```python
from build123d import *

# Parameters (mm, degrees)
SKIZZE1_W                                      = 100
SKIZZE1_H                                      = 70
SKIZZE1_W_2                                    = 55
SKIZZE1_H_2                                    = 10
AUFSATZ_LINEAR_AUSTRAGEN1_DEPTH                = 2
F_3_5_3_5_DURCHMESSER_BOHRUNG1_D               = 3.5
FORMSENKUNG_F_R_M3_LINSENSENKSCHRAUB_2_COUNT   = 2
FORMSENKUNG_F_R_M3_LINSENSENKSCHRAUB_2_PITCH   = 90
FORMSENKUNG_F_R_M3_LINSENSENKSCHRAUB_3_COUNT   = 2
FORMSENKUNG_F_R_M3_LINSENSENKSCHRAUB_3_PITCH   = 108.166538264
FORMSENKUNG_F_R_M3_LINSENSENKSCHRAUB_4_COUNT   = 2
FORMSENKUNG_F_R_M3_LINSENSENKSCHRAUB_4_PITCH   = 60
FORMSENKUNG_F_R_M3_LINSENSENKSCHRAUB_5_A_COUNT = 2
FORMSENKUNG_F_R_M3_LINSENSENKSCHRAUB_5_A_PITCH = 20


with BuildPart() as part:
    # Skizze1 → Aufsatz-Linear austragen1 (new body)
    with BuildSketch(Plane(origin=(0, 0, 0), x_dir=(1, 0, 0), z_dir=(0, 1, 0))):
        with Locations((50, 35)):
            Rectangle(SKIZZE1_W, SKIZZE1_H)
        with Locations((37.5, 55)):
            Rectangle(SKIZZE1_W_2, SKIZZE1_H_2, mode=Mode.SUBTRACT)
    extrude(amount=AUFSATZ_LINEAR_AUSTRAGEN1_DEPTH)

    # Ø3.5 (3.5) Durchmesser Bohrung1 (through all)
    with Locations(Plane(origin=(0, 2, 0), x_dir=(1, 0, 0), z_dir=(0, 1, 0))):
        with Locations((7, 55), (68, 55)):
            Hole(F_3_5_3_5_DURCHMESSER_BOHRUNG1_D / 2)

    # Skizze7 → Formsenkung f_r M3 Linsensenkschraube mi (revolve, cut)
    with BuildSketch(Plane(origin=(5, 0, -5), x_dir=(0, 0, -1), z_dir=(1, 0, 0))):
        Polygon((0, 0), (0, 2), (1.725, 2), (1.7, 1.975), (1.7, 1.45), (3.15, 0), align=None)
    formsenkung_f_r_m3_linsensenkschraube_mi = revolve(axis=Axis((5, -6.35, -5), (0, 1, 0)), mode=Mode.SUBTRACT)

    # Formsenkung f_r M3 Linsensenkschraub 2: Formsenkung f_r M3 Linsensenkschraube mi ×2
    with Locations(*[(i * FORMSENKUNG_F_R_M3_LINSENSENKSCHRAUB_2_PITCH, 0, 0) for i in range(1, FORMSENKUNG_F_R_M3_LINSENSENKSCHRAUB_2_COUNT)]):
        add(formsenkung_f_r_m3_linsensenkschraube_mi, mode=Mode.SUBTRACT)

    # Formsenkung f_r M3 Linsensenkschraub 3: Formsenkung f_r M3 Linsensenkschraube mi ×2
    with Locations(*[Vector(0.8320502943378437, 0, -0.5547001962252291) * (i * FORMSENKUNG_F_R_M3_LINSENSENKSCHRAUB_3_PITCH) for i in range(1, FORMSENKUNG_F_R_M3_LINSENSENKSCHRAUB_3_COUNT)]):
        add(formsenkung_f_r_m3_linsensenkschraube_mi, mode=Mode.SUBTRACT)

    # Formsenkung f_r M3 Linsensenkschraub 4: Formsenkung f_r M3 Linsensenkschraube mi ×2
    with Locations(*[(0, 0, -i * FORMSENKUNG_F_R_M3_LINSENSENKSCHRAUB_4_PITCH) for i in range(1, FORMSENKUNG_F_R_M3_LINSENSENKSCHRAUB_4_COUNT)]):
        add(formsenkung_f_r_m3_linsensenkschraube_mi, mode=Mode.SUBTRACT)

    # Skizze9 → Formsenkung f_r M3 Linsensenkschraub 5 (revolve, cut)
    with BuildSketch(Plane(origin=(85, 0, -10), x_dir=(0, 0, -1), z_dir=(1, 0, 0))):
        Polygon((0, 0), (0, 2), (1.725, 2), (1.7, 1.975), (1.7, 1.45), (3.15, 0), align=None)
    formsenkung_f_r_m3_linsensenkschraub_5 = revolve(axis=Axis((85, -6.35, -10), (0, 1, 0)), mode=Mode.SUBTRACT)

    # Formsenkung f_r M3 Linsensenkschraub 5 a: Formsenkung f_r M3 Linsensenkschraub 5 ×2
    with Locations(*[(0, 0, -i * FORMSENKUNG_F_R_M3_LINSENSENKSCHRAUB_5_A_PITCH) for i in range(1, FORMSENKUNG_F_R_M3_LINSENSENKSCHRAUB_5_A_COUNT)]):
        add(formsenkung_f_r_m3_linsensenkschraub_5, mode=Mode.SUBTRACT)


solid = part.part
```
Input: part model. Units: mm. Frame: model coordinates. A direction names the side the tool comes from. Give positions to 0.01 mm unless a question says otherwise; leave off trailing zeros. Loops run counter-clockwise (first coordinate to the right, second up) from the corner with the lowest first, then second, coordinate; pieces in that order, holes last. Notation, with made-up numbers: M 17,36 L 76,36 A14 cw 76,63 Z; hole C 41,-33.75 d1. An arc over 180 degrees is marked long. Answer as CSV lines item,"result". Start each with the question number.
1. Reachability of faces 4 (the face through (37, 1, -50)), 5 (the face through (0, 1, -35)) from +Z, -Z, +X, -X, +Y, -Y: full face, straight path, thin tool, end or side. Return the list, or none.
2. Section B-B on z = -65. Return loops of the section in (x, y) (3 decimals), plus the area to 3 significant figures.
3. Section D-D on x = 85. Return loops of the section in (y, z) (3 decimals).
4. Line query: L1, parallel to Z at x = 85, y = 1.7; L2, parallel to X at y = 1.7, z = -5; L3, parallel to Z at x = 60.5, y = 1.65. Output: solid intervals per line, ascending.
5. Pull-direction query (Z, two-part tool) for faces 1 (the face through (49, 1, -70)), 2 (the face through (49, 1, 0)), 3 (the face through (4.93, 1.71, -63.3)); classes: released by +Z, released by -Z, zero draft, split by the parting line, or undercut.
6. Section C-C on x = 55.5. Return loops of the section in (y, z), plus the area to 3 significant figures.
7. Section A-A on z = -10. Return loops of the section in (x, y) (3 decimals).
8. Pin query (flat end, axial travel): P1, Ø4, axis at x = 95, z = -5, coming from the -Y side. Return the tip coordinate at first contact, or that it passes through.
Computed values:
1,face 4,"+Y, -Y"
1,face 5,"+Z, -Z, -X, +Y, -Y"
2,outline,"M 0,0 L 1.85,0 L 3.3,1.45 L 3.3,1.975 L 3.275,2 L 0,2 Z; M 6.7,1.45 L 8.15,0 L 91.85,0 L 93.3,1.45 L 93.3,1.975 L 93.275,2 L 6.725,2 L 6.7,1.975 Z; M 96.7,1.45 L 98.15,0 L 100,0 L 100,2 L 96.725,2 L 96.7,1.975 Z"
2,area,"182 mm²"
3,outline,"M 0,-70 L 2,-70 L 2,-31.725 L 1.975,-31.7 L 1.45,-31.7 L 0,-33.15 Z; M 0,-26.85 L 1.45,-28.3 L 1.975,-28.3 L 2,-28.275 L 2,-11.725 L 1.975,-11.7 L 1.45,-11.7 L 0,-13.15 Z; M 0,-6.85 L 1.45,-8.3 L 1.975,-8.3 L 2,-8.275 L 2,0 L 0,0 Z"
4,L1,"z = -70 to -31.7, -28.3 to -11.7, -8.3 to 0"
4,L2,"x = 0 to 3.3, 6.7 to 93.3, 96.7 to 100"
4,L3,"z = -70 to -60, -50 to 0"
5,face 1,"released by -Z"
5,face 2,"released by +Z"
5,face 3,"undercut"
6,outline,"M 0,-70 L 2,-70 L 2,-60 L 0,-60 Z; M 0,-50 L 2,-50 L 2,0 L 0,0 Z"
6,area,"120 mm²"
7,outline,"M 0,0 L 81.85,0 L 83.3,1.45 L 83.3,1.975 L 83.275,2 L 0,2 Z; M 86.7,1.45 L 88.15,0 L 100,0 L 100,2 L 86.725,2 L 86.7,1.975 Z"
8,P1,"stops at y = 1.15"
